from build123d import *

# Parameters (mm, degrees)
SKETCH1_W                     = 304.8
SKETCH1_H                     = 86.36
BOSS_EXTRUDE1_DEPTH           = 1.5875
F_4_CLEARANCE_HOLE1_OUTLINE_R = 1.4732
F_4_CLEARANCE_HOLE1_DEPTH     = 1.5875
F_1_8_0_125_DIAMETER_HOLE1_D  = 3.175
CUT_EXTRUDE1_DEPTH            = 317.802161855
F_4_CLEARANCE_HOLE2_D         = 2.9464
F_4_CLEARANCE_HOLE2_DEPTH     = 9.1694
F_4_CLEARANCE_HOLE2_TIP       = 0.885187864
CUT_EXTRUDE3_DEPTH            = 317.802161855
F_4_CLEARANCE_HOLE3_D         = 2.9464
F_4_CLEARANCE_HOLE3_DEPTH     = 9.1694
F_4_CLEARANCE_HOLE3_TIP       = 0.885187864


# Read off the part's stored shape, not the designer's step: #4 Clearance Hole1
with BuildPart() as part:
    # Sketch1 → Boss-Extrude1 (new body)
    with BuildSketch(Plane(origin=(0, 0, 0), x_dir=(0, 0, -1), z_dir=(1, 0, 0))):
        with Locations((152.4, 43.18)):
            Rectangle(SKETCH1_W, SKETCH1_H)
    extrude(amount=BOSS_EXTRUDE1_DEPTH)

    # #4 Clearance Hole1 outline → #4 Clearance Hole1 (cut)
    with BuildSketch(Plane.YZ):
        with Locations((68.36, -269.24)):
            Circle(F_4_CLEARANCE_HOLE1_OUTLINE_R)
        with Locations((18, -269.24)):
            Circle(F_4_CLEARANCE_HOLE1_OUTLINE_R)
        with Locations((82.55, -25.4)):
            Circle(F_4_CLEARANCE_HOLE1_OUTLINE_R)
        with Locations((82.55, -88.9)):
            Circle(F_4_CLEARANCE_HOLE1_OUTLINE_R)
        with Locations((82.55, -190.5)):
            Circle(F_4_CLEARANCE_HOLE1_OUTLINE_R)
        with Locations((82.55, -254)):
            Circle(F_4_CLEARANCE_HOLE1_OUTLINE_R)
        with Locations((3.81, -254)):
            Circle(F_4_CLEARANCE_HOLE1_OUTLINE_R)
        with Locations((3.81, -190.5)):
            Circle(F_4_CLEARANCE_HOLE1_OUTLINE_R)
        with Locations((3.81, -88.9)):
            Circle(F_4_CLEARANCE_HOLE1_OUTLINE_R)
        with Locations((3.81, -25.4)):
            Circle(F_4_CLEARANCE_HOLE1_OUTLINE_R)
    extrude(amount=F_4_CLEARANCE_HOLE1_DEPTH, mode=Mode.SUBTRACT)

    # 1/8 (0.125) Diameter Hole1 (through all)
    with Locations(Plane(origin=(1.5875, 0, 0), x_dir=(0, 0, -1), z_dir=(1, 0, 0))):
        with Locations((278.8359549, 43.18)):
            Hole(F_1_8_0_125_DIAMETER_HOLE1_D / 2)

    # Sketch6 → Cut-Extrude1 (cut, through all)
    with BuildSketch(Plane(origin=(1.5875, 0, 0), x_dir=(0, 0, -1), z_dir=(1, 0, 0))):
        with BuildLine():
            Line((141.5288, 60.96), (141.5288, 48.26))
            ThreePointArc((141.5288, 48.26), (139.7, 46.4312), (137.8712, 48.26))
            Line((137.8712, 48.26), (137.8712, 60.96))
            ThreePointArc((137.8712, 60.96), (139.7, 62.7888), (141.5288, 60.96))
        make_face()
        with BuildLine():
            Line((141.5288, 25.4), (141.5288, 38.1))
            ThreePointArc((141.5288, 38.1), (139.7, 39.9288), (137.8712, 38.1))
            Line((137.8712, 38.1), (137.8712, 25.4))
            ThreePointArc((137.8712, 25.4), (139.7, 23.5712), (141.5288, 25.4))
        make_face()
    extrude(amount=-CUT_EXTRUDE1_DEPTH, mode=Mode.SUBTRACT)

    # #4 Clearance Hole2
    with Locations(Plane.ZY):
        with Locations((-228.6, 5.1562), (-228.6, 81.2038), (-172.72, 5.1562), (-172.72, 81.2038), (-106.68, 5.1562), (-50.8, 5.1562), (-106.68, 81.2038), (-50.8, 81.2038)):
            Hole(F_4_CLEARANCE_HOLE2_D / 2, depth=F_4_CLEARANCE_HOLE2_DEPTH)
            with Locations((0, 0, -(F_4_CLEARANCE_HOLE2_DEPTH + F_4_CLEARANCE_HOLE2_TIP / 2))):  # 118° drill point
                Cone(0, F_4_CLEARANCE_HOLE2_D / 2, F_4_CLEARANCE_HOLE2_TIP, mode=Mode.SUBTRACT)

    # Sketch10 → Cut-Extrude3 (cut, through all)
    with BuildSketch(Plane.ZY):
        with BuildLine():
            Line((-100.33, 49.53), (-74.93, 49.53))
            ThreePointArc((-74.93, 49.53), (-68.58, 43.18), (-74.93, 36.83))
            Line((-74.93, 36.83), (-100.33, 36.83))
            ThreePointArc((-100.33, 36.83), (-106.68, 43.18), (-100.33, 49.53))
        make_face()
    extrude(amount=-CUT_EXTRUDE3_DEPTH, mode=Mode.SUBTRACT)

    # #4 Clearance Hole3
    with Locations(Plane.ZY):
        with Locations((-6.35, 12.7), (-6.35, 73.66), (-298.45, 12.7), (-298.45, 73.66)):
            Hole(F_4_CLEARANCE_HOLE3_D / 2, depth=F_4_CLEARANCE_HOLE3_DEPTH)
            with Locations((0, 0, -(F_4_CLEARANCE_HOLE3_DEPTH + F_4_CLEARANCE_HOLE3_TIP / 2))):  # 118° drill point
                Cone(0, F_4_CLEARANCE_HOLE3_D / 2, F_4_CLEARANCE_HOLE3_TIP, mode=Mode.SUBTRACT)


solid = part.part
Verification items for the finished model (mm, model axes). A direction names the side the tool comes from. Give positions to 0.01 mm unless a question says otherwise; leave off trailing zeros.
1) Depth check by flat-ended pin: pin 1 Ø3.5 at (y, z) = (12.7, -6.35) entering from +X; pin 2 Ø2.5 at (y, z) = (82.55, -254) entering from +X. Enter the tip coordinate at first touch or a pass-through.
2) Thickness scan on line 1 along Y through (x, z) = (0.75, -88.9); line 2 along Y through (x, z) = (1.05, -269.24); line 3 along Z through (x, y) = (1.5, 26.5). Record the ranges inside material, lowest first.
3) Sectioned sample at A-A, the plane x = 1.25. Count the separate pieces of the cut face and the enclosed holes in it, then the cut area to 3 significant figures.
4) Draft check along Z on faces 3 (the cylindrical face through (0.78, 43.04, -106.68)), 4 (the flat face through (0, 44, -150)). Enter one of: pulls with the +Z half, pulls with the -Z half, needs draft (parallel to the pull), parting line crosses it, or undercut.
5) Set-up check for faces 1 (the cylindrical face through (0.78, 43.32, -68.58)), 2 (the flat face through (1.588, 44, -150)): record each of +Z, -Z, +X, -X, +Y, -Y from which the full face is reachable in a straight line by a thin tool's end or side.
Answers:
1. pin 1: stops at x = 1.59
1. pin 2: passes through
2. line 1: y = 0 to 2.34, 5.28 to 36.83, 49.53 to 81.08, 84.02 to 86.36
2. line 2: y = 0 to 16.53, 19.47 to 66.89, 69.83 to 86.36
2. line 3: z = -304.8 to -141.53, -137.87 to 0
3. separate pieces: 1
3. enclosed holes: 26
3. area: 25,600 mm2
4. face 3: undercut
4. face 4: needs draft
5. face 1: +X, -X
5. face 2: +Z, -Z, +X, +Y, -Y
